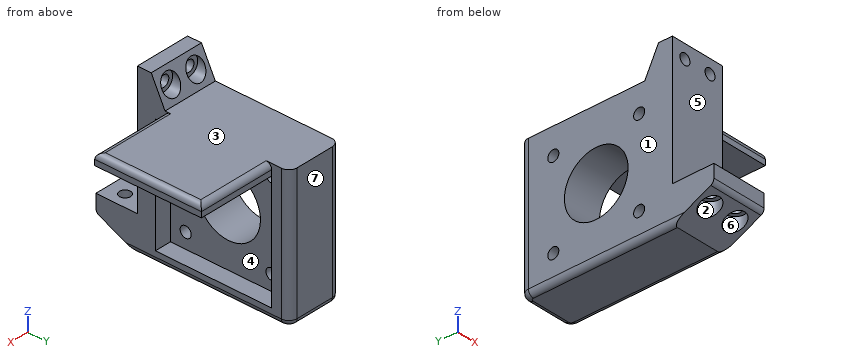
from build123d import *

# Parameters (mm, degrees)
SKETCH1_W           = 20
SKETCH1_H           = 50
BOSS_EXTRUDE1_DEPTH = 70
SKETCH2_R           = 2
SKETCH2_R_2         = 11.5
CUT_EXTRUDE2_DEPTH  = 60
SKETCH4_W           = 37
SKETCH4_H           = 15
CUT_EXTRUDE3_DEPTH  = 60
SKETCH8_R           = 2
CUT_EXTRUDE5_DEPTH  = 15
SKETCH9_W           = 42
SKETCH9_H           = 42
CUT_EXTRUDE6_DEPTH  = 6
CUT_EXTRUDE8_DEPTH  = 30
SKETCH12_W          = 20
SKETCH12_H          = 5
BOSS_EXTRUDE2_DEPTH = 10
BOSS_EXTRUDE3_DEPTH = 20
SKETCH15_R          = 2
CUT_EXTRUDE9_DEPTH  = 10
SKETCH17_R          = 3.5
CUT_EXTRUDE11_DEPTH = 8
SKETCH18_R          = 3.5
CUT_EXTRUDE12_DEPTH = 50
FILLET2_R           = 3
FILLET3_R           = 3
FILLET5_R           = 2
FILLET6_R           = 2
SKETCH19_W          = 4
SKETCH19_H          = 38.5
BOSS_EXTRUDE4_DEPTH = 28
FILLET7_R           = 2


with BuildPart() as part:
    # Sketch1 → Boss-Extrude1 (new body)
    with BuildSketch(Plane(origin=(0, 0, 0), x_dir=(1, 0, 0), z_dir=(0, 1, 0))):
        with Locations((-10, -25)):
            Rectangle(SKETCH1_W, SKETCH1_H)
    extrude(amount=BOSS_EXTRUDE1_DEPTH)

    # Sketch2 → Cut-Extrude2 (cut)
    with BuildSketch(Plane(origin=(0, 0, 0), x_dir=(0, 0, -1), z_dir=(1, 0, 0))):
        with Locations((-9.5, 58)):
            Circle(SKETCH2_R)
        with Locations((-25, 42.5)):
            Circle(SKETCH2_R_2)
        with Locations((-9.5, 27)):
            Circle(SKETCH2_R)
        with Locations((-40.5, 27)):
            Circle(SKETCH2_R)
        with Locations((-40.5, 58)):
            Circle(SKETCH2_R)
    extrude(amount=-CUT_EXTRUDE2_DEPTH, mode=Mode.SUBTRACT)

    # Sketch4 → Cut-Extrude3 (cut)
    with BuildSketch(Plane(origin=(0, 0, 0), x_dir=(0, 0, -1), z_dir=(1, 0, 0))):
        with Locations((-31.5, 7.5)):
            Rectangle(SKETCH4_W, SKETCH4_H)
    extrude(amount=-CUT_EXTRUDE3_DEPTH, mode=Mode.SUBTRACT)

    # Sketch8 → Cut-Extrude5 (cut)
    with BuildSketch(Plane(origin=(0, 0, 0), x_dir=(-1, 0, 0), z_dir=(0, 0, -1))):
        with Locations((15, 6)):
            Circle(SKETCH8_R)
        with Locations((5, 6)):
            Circle(SKETCH8_R)
    extrude(amount=-CUT_EXTRUDE5_DEPTH, mode=Mode.SUBTRACT)

    # Sketch9 → Cut-Extrude6 (cut)
    with BuildSketch(Plane(origin=(0, 0, 0), x_dir=(0, 0, -1), z_dir=(1, 0, 0))):
        with Locations((-25, 42.5)):
            Rectangle(SKETCH9_W, SKETCH9_H)
    extrude(amount=-CUT_EXTRUDE6_DEPTH, mode=Mode.SUBTRACT)

    # Sketch11 → Cut-Extrude8 (cut)
    with BuildSketch(Plane(origin=(0, 0, 0), x_dir=(0, 0, -1), z_dir=(1, 0, 0))):
        Polygon((-7, 0), (0, 0), (0, 15), align=None)
    extrude(amount=-CUT_EXTRUDE8_DEPTH, mode=Mode.SUBTRACT)

    # Sketch12 → Boss-Extrude2 (add)
    with BuildSketch(Plane.XY.offset(50)):
        with Locations((-10, 17.5)):
            Rectangle(SKETCH12_W, SKETCH12_H)
    extrude(amount=BOSS_EXTRUDE2_DEPTH)

    # Sketch14 → Boss-Extrude3 (add)
    with BuildSketch(Plane(origin=(0, 0, 0), x_dir=(0, 0, -1), z_dir=(1, 0, 0))):
        Polygon((-50, 20), (-60, 20), (-50, 25), align=None)
    extrude(amount=-BOSS_EXTRUDE3_DEPTH)

    # Sketch15 → Cut-Extrude9 (cut)
    with BuildSketch(Plane(origin=(0, 15, 0), x_dir=(-1, 0, 0), z_dir=(0, -1, 0))):
        with Locations(Location((5, -55, 0), (0, 0, 90))):
            Circle(SKETCH15_R)
        with Locations(Location((15, -55, 0), (0, 0, 90))):
            Circle(SKETCH15_R)
    extrude(amount=-CUT_EXTRUDE9_DEPTH, mode=Mode.SUBTRACT)

    # Sketch17 → Cut-Extrude11 (cut)
    with BuildSketch(Plane(origin=(0, 0, 0), x_dir=(-1, 0, 0), z_dir=(0, 0, -1))):
        with Locations((15, 6)):
            Circle(SKETCH17_R)
        with Locations((5, 6)):
            Circle(SKETCH17_R)
    extrude(amount=-CUT_EXTRUDE11_DEPTH, mode=Mode.SUBTRACT)

    # Sketch18 → Cut-Extrude12 (cut)
    with BuildSketch(Plane(origin=(0, 70, 0), x_dir=(1, 0, 0), z_dir=(0, 1, 0))):
        with Locations(Location((-15, -55, 0), (0, 0, 270))):
            Circle(SKETCH18_R)
        with Locations(Location((-5, -55, 0), (0, 0, 270))):
            Circle(SKETCH18_R)
    extrude(amount=-CUT_EXTRUDE12_DEPTH, mode=Mode.SUBTRACT)

    # Fillet2
    fillet2_edges = [part.edges().sort_by_distance(p)[0] for p in [
        (0, 70, 25),
    ]]
    fillet(fillet2_edges, radius=FILLET2_R)

    # Fillet3
    fillet3_edges = [part.edges().sort_by_distance(p)[0] for p in [
        (-20, 70, 25),
    ]]
    fillet(fillet3_edges, radius=FILLET3_R)

    # Fillet5
    fillet5_edges = [part.edges().sort_by_distance(p)[0] for p in [
        (-10, 70, 0),
        (0, 41, 0),
        (-0.878679656, 69.121320344, 0),
        (-20, 41, 0),
        (-19.121320344, 69.121320344, 0),
    ]]
    fillet(fillet5_edges, radius=FILLET5_R)

    # Fillet6
    fillet6_edges = [part.edges().sort_by_distance(p)[0] for p in [
        (-10, 0, 7),
    ]]
    fillet(fillet6_edges, radius=FILLET6_R)

    # Sketch19 → Boss-Extrude4 (add)
    with BuildSketch(Plane(origin=(0, 0, 0), x_dir=(0, 0, -1), z_dir=(1, 0, 0))):
        with Locations((-48, 44.25)):
            Rectangle(SKETCH19_W, SKETCH19_H)
    extrude(amount=BOSS_EXTRUDE4_DEPTH)

    # Fillet7
    fillet7_edges = [part.edges().sort_by_distance(p)[0] for p in [
        (14, 63.5, 50),
        (14, 25, 50),
        (28, 44.25, 50),
    ]]
    fillet(fillet7_edges, radius=FILLET7_R)


solid = part.part
Work out the finished part from the listing and answer in its coordinate system (mm). Face numbers are marked on the shaded views. A direction names the side the tool comes from. Coordinates: 2 decimals unless noted, no trailing zeros. Write each loop counter-clockwise with the first axis right and the second up, starting at its lowest first coordinate (ties: lowest second). Pieces come first, ordered by that corner, then holes. Notation, with made-up numbers: M 41.25,-20 L 51.25,-20 A11 ccw 51.25,-16 Z; hole C 81.25,56.5 d10. An arc over 180 degrees is marked long. Write item = value, one per line.
1. The part is cut by section A-A (z = 9.5). Determine the outline of the cut face in (x, y).
Solution:
outline = M -20,0 L 0,0 L 0,21.5 L -6,21.5 L -6,25 L -20,25 Z; M -20,29 L -6,29 L -6,56 L -20,56 Z; M -20,60 L -6,60 L -6,63.5 L 0,63.5 L 0,67 A3 ccw -3,70 L -17,70 A3 ccw -20,67 Z; hole C -15,6 d4; hole C -5,6 d4
2. The part is cut by section C-C (z = 55). Determine the outline of the cut face in (x, y), then the cut area to 3 significant figures.
Solution:
outline = M -20,15 L -17,15 L -17,20 L -18.5,20 L -18.5,22.5 L -20,22.5 Z; M -13,15 L -7,15 L -7,20 L -8.5,20 L -8.5,22.5 L -11.5,22.5 L -11.5,20 L -13,20 Z; M -3,15 L 0,15 L 0,22.5 L -1.5,22.5 L -1.5,20 L -3,20 Z
area = 75.0 mm2
3. Determine the mould class of the marked faces 1, 2 and 3 for opening direction X: released by +X, released by -X, zero draft, split by the parting line, or undercut.
Solution:
face_1 = released by -X
face_2 = undercut
face_3 = zero draft
4. Straight lines are drawn through the part: line 1 (X direction, y = 18.25, z = 55); line 2 (X direction, y = 6, z = 6.7); line 3 (Y direction, x = -8.75, z = 9.5). For each, find the intervals that lie inside material, in ascending order. Write a range as from..to.
Solution:
line_1 = -20..-17, -13..-7, -3..0
line_2 = -20..-18.5, -11.5..-8.5, -1.5..0
line_3 = 0..25, 29..56, 60..70
5. The part is cut by section D-D (y = 17.5). Determine the outline of the cut face in (x, z).
Solution:
outline = M -20,2 A2 ccw -18,0 L -2,0 A2 ccw 0,2 L 0,60 L -20,60 Z; hole C -15,55 d4; hole C -5,55 d4
6. The part is cut by section B-B (y = 42.5). Determine the outline of the cut face in (x, z).
Solution:
outline = M -20,2 A2 ccw -18,0 L -2,0 A2 ccw 0,2 L 0,4 L -6,4 L -6,13.5 L -20,13.5 Z; M -20,36.5 L -6,36.5 L -6,46 L 28,46 L 28,48 A2 ccw 26,50 L -20,50 Z
7. Flat-ended cylindrical pins translate along their axes: pin 1 (3 mm diameter, centred on y = 27, z = 9.5, fed in from -X); pin 2 (8 mm diameter, centred on x = 11.5, y = 61.5, fed in from +Z); pin 3 (8 mm diameter, centred on x = -15, z = 55, fed in from +Y); pin 4 (8 mm diameter, centred on x = 12.5, y = 24.5, fed in from -Z). Find the tip coordinate at first contact, or state that the pin passes through.
Solution:
pin_1 = through
pin_2 = 50
pin_3 = 24.5
pin_4 = 46
8. For the marked faces 4, 5, 6 and 7, determine the directions among +Z, -Z, +X, -X, +Y, -Y from which every point of the face is accessible in a straight line to the end or side of a thin tool.
Solution:
face_4 = +X
face_5 = +Z, +X, -X, -Y
face_6 = -Z
face_7 = +Z, -Z, +X, -X, +Y
